```python
from build123d import *

# Parameters (mm, degrees)
F0_W      = 104.71709
F0_H      = 61.959744
F1_DEPTH  = 16.002
F2_R      = 23.822659
F2_R_2    = 17.472659
F3_DEPTH  = 25.4
F3_FACE_R = 17.472659
F4_DEPTH  = 25.4


with BuildPart() as f1:
    # F0 (on Top) → F1 (new body)
    with BuildSketch(Plane.XY):
        Rectangle(F0_W, F0_H)
    extrude(amount=F1_DEPTH)

    # F2 (on face) → F3 (join)
    with BuildSketch(Plane.XY.offset(16.002)):
        Circle(F2_R)
        Circle(F2_R_2, mode=Mode.SUBTRACT)
    extrude(amount=F3_DEPTH)

    # F3_face (on face) → F4 (cut)
    with BuildSketch(Plane.XY.offset(16.002)):
        Circle(F3_FACE_R)
    extrude(amount=-F4_DEPTH, mode=Mode.SUBTRACT)


solid = f1.part
```
CAD build for the part. Positions are in the model's coordinates, mm. A direction names the side the tool comes from. Coordinates: 2 decimals unless noted, no trailing zeros. Write each loop counter-clockwise with the first axis right and the second up, starting at its lowest first coordinate (ties: lowest second). Pieces come first, ordered by that corner, then holes.
(1) Drill centre lines: probe 1 along Y at (x, z) = (0, 5.75); probe 2 along Y at (x, z) = (0, 23); probe 3 along X at (y, z) = (-3, 17). Where is each one in solid material? Low to high.
(2) Cut at A-A, the plane x = 0. List the corners of the cut face in (y, z), and give its area (3 significant figures).
(3) Cut at D-D, the plane x = 22. List the corners of the cut face in (y, z), and give its area (3 significant figures).
(4) Cut at B-B, the plane y = 0. List the corners of the cut face in (x, z).
(5) Flat gauge pin, fed straight in: pin 1 (5 mm diameter, centred on x = -30.5, y = 17.5, fed in from +Z). Where does the tip first touch, or does it go through?
(6) Cut at C-C, the plane z = 5. List the corners of the cut face in (x, y).
(7) 3-axis set-ups, long thin cutter, end or side, ignore diameter. For faces 1 (the face through (-5.164, -23.256, 28.524)), 2 (the face through (-12, 14, 0)): which of +Z, -Z, +X, -X, +Y, -Y reach the whole face in a straight line?
Geometry says:
1. probe 1: y = -30.98 to -17.47, 17.47 to 30.98
1. probe 2: y = -23.82 to -17.47, 17.47 to 23.82
1. probe 3: x = -23.63 to -17.21, 17.21 to 23.63
2. outline: (-30.98, 0) - (-17.47, 0) - (-17.47, 41.4) - (-23.82, 41.4) - (-23.82, 16) - (-30.98, 16) - close; (17.47, 0) - (30.98, 0) - (30.98, 16) - (23.82, 16) - (23.82, 41.4) - (17.47, 41.4) - close
2. area: 755 mm2
3. outline: (-30.98, 0) - (30.98, 0) - (30.98, 16) - (9.14, 16) - (9.14, 41.4) - (-9.14, 41.4) - (-9.14, 16) - (-30.98, 16) - close
3. area: 1,460 mm2
4. outline: (-52.36, 0) - (-17.47, 0) - (-17.47, 41.4) - (-23.82, 41.4) - (-23.82, 16) - (-52.36, 16) - close; (17.47, 0) - (52.36, 0) - (52.36, 16) - (23.82, 16) - (23.82, 41.4) - (17.47, 41.4) - close
5. pin 1: stops at z = 16
6. outline: (-52.36, -30.98) - (52.36, -30.98) - (52.36, 30.98) - (-52.36, 30.98) - close; hole circle Ø34.95 at (0, 0)
7. face 1: +Z
7. face 2: -Z, +X, -X, +Y, -Y
